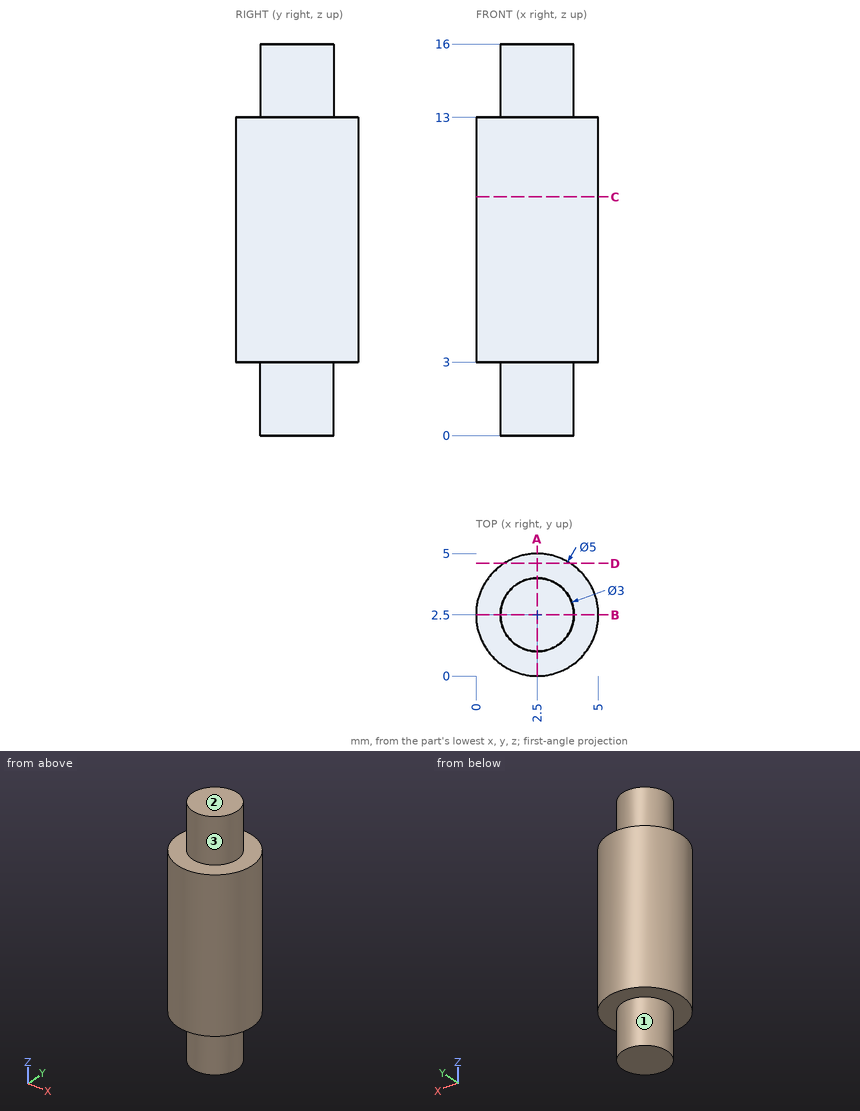
Check sheet for the drawn part. Datum: minimum x, y, z corner. Units: mm. A direction names the side the tool comes from. Give positions to 0.01 mm unless a question says otherwise; leave off trailing zeros. Write each loop counter-clockwise with the first axis right and the second up, starting at its lowest first coordinate (ties: lowest second). Pieces come first, ordered by that corner, then holes.
(1) Gauge pin test, flat end, axial feed: pin 1 (1 mm diameter, centred on x = 3.5, y = 2.5, fed in from -Z). Record the tip position at first contact, or that the pin passes through.
(2) Access from +Z, -Z, +X, -X, +Y, -Y to the whole of each face (thin tool, end or side, straight path). Record for the marked faces 1, 2 and 3.
(3) Cross-section at D-D (y = 4.6). Enter the section's corners in (x, z), plus the area to 3 significant figures.
(4) Cross-section at C-C (z = 9.75). Enter the section's corners in (x, y), plus the area to 3 significant figures.
(5) Material ranges on line 1 (Z direction, x = 3.75, y = 3.75); line 2 (X direction, y = 2.6, z = 10); line 3 (Y direction, x = 0.5, z = 12), recorded low to high.
(6) Cross-section at A-A (x = 2.5). Enter the section's corners in (y, z), plus the area to 3 significant figures.
Worked out:
1. pin 1: stops at z = 0
2. face 1: -Z
2. face 2: +Z, +X, -X, +Y, -Y
2. face 3: +Z
3. outline: (1.14, 3) - (3.86, 3) - (3.86, 13) - (1.14, 13) - close
3. area: 27.1 mm2
4. outline: circle Ø5 at (2.5, 2.5)
4. area: 19.6 mm2
5. line 1: z = 3 to 13
5. line 2: x = 0 to 5
5. line 3: y = 1 to 4
6. outline: (0, 3) - (1, 3) - (1, 0) - (4, 0) - (4, 3) - (5, 3) - (5, 13) - (4, 13) - (4, 16) - (1, 16) - (1, 13) - (0, 13) - close
6. area: 68.0 mm2
